Can you work these out from the model? Positions are in its coordinate system, mm. Face numbers are marked on the shaded views. A direction names the side the tool comes from. Coordinates: 2 decimals unless noted, no trailing zeros. Loops run counter-clockwise (first coordinate to the right, second up) from the corner with the lowest first, then second, coordinate; pieces in that order, holes last. Notation, with made-up numbers: M 12.25,75 L 57.25,75 A17 cw 57.25,85 Z; hole C 35,54.25 d8. An arc over 180 degrees is marked long. Answer as a JSON object with one key per item and string values. Group by question number.
Item 1: I'm going to push a flat-ended pin straight in: pin 1 Ø5 at (y, z) = (-1.5, 12) entering from +X. Where does the tip first touch, or does it pass through?
Item 2: Which directions (+Z, -Z, +X, -X, +Y, -Y) give clear straight access to the entire face, cutting with the end or side of a thin tool? Please do the marked faces 4 and 5.
Item 3: We'd pull the mould along Y, two halves only. Please class the marked faces 1, 2 and 3: +Y half, -Y half, draft (parallel to the pull), parting line (faces both ways), or undercut.
Item 4: Suppose I cut it at A-A (x = -7.5). Write out the boundary of the cut face in (y, z).
Item 5: If I drill on line 1 (X direction, y = -7, z = 3); line 2 (Y direction, x = 4.5, z = 46), over which ranges is the centre line in solid material (lowest first)?
```python
from build123d import *

# Parameters (mm, degrees)
RESSALTO_EXTRUS_O1_DEPTH = 50
PADR_OCIRCULAR1_COUNT    = 4
FILETE1_R                = 0.4


with BuildPart() as part:
    # Esboço1 → Ressalto-extrusão1 (new body)
    with BuildSketch(Plane.XY):
        with BuildLine():
            ThreePointArc((-9.317157288, 3.217157288), (-9.187387948, 3.130448187), (-9.034314575, 3.1))
            Line((-9.034314575, 3.1), (-8.9, 3.1))
            ThreePointArc((-8.9, 3.1), (-8.617157288, 3.217157288), (-8.5, 3.5))
            Line((-8.5, 3.5), (-8.5, 5.5))
            Line((-8.5, 5.5), (-6.560660172, 5.5))
            Line((-6.560660172, 5.5), (-5.064466094, 4.003805922))
            ThreePointArc((-5.064466094, 4.003805922), (-3.980602337, 2.381689178), (-3.6, 0.468272016))
            Line((-3.6, 0.468272016), (-3.6, 0))
            Line((-3.6, 0), (-2.5, 0))
            ThreePointArc((-2.5, 0), (-1.767766953, 1.767766953), (0, 2.5))
            Line((0, 2.5), (0, 3.6))
            Line((0, 3.6), (-0.468272016, 3.6))
            ThreePointArc((-0.468272016, 3.6), (-2.381689178, 3.980602337), (-4.003805922, 5.064466094))
            Line((-4.003805922, 5.064466094), (-5.5, 6.560660172))
            Line((-5.5, 6.560660172), (-5.5, 8.5))
            Line((-5.5, 8.5), (-3.5, 8.5))
            ThreePointArc((-3.5, 8.5), (-3.217157288, 8.617157288), (-3.1, 8.9))
            Line((-3.1, 8.9), (-3.1, 9.034314575))
            ThreePointArc((-3.1, 9.034314575), (-3.130448187, 9.187387948), (-3.217157288, 9.317157288))
            Line((-3.217157288, 9.317157288), (-3.782842712, 9.882842712))
            ThreePointArc((-3.782842712, 9.882842712), (-3.912612052, 9.969551813), (-4.065685425, 10))
            Line((-4.065685425, 10), (-10, 10))
            Line((-10, 10), (-10, 4.065685425))
            ThreePointArc((-10, 4.065685425), (-9.969551813, 3.912612052), (-9.882842712, 3.782842712))
            Line((-9.882842712, 3.782842712), (-9.317157288, 3.217157288))
        make_face()
    ressalto_extrus_o1 = extrude(amount=RESSALTO_EXTRUS_O1_DEPTH)

    # PadrãoCircular1: Ressalto-extrusão1 ×4 about axis
    padr_ocircular1_axis = Axis((0, 0, 0), (0, 0, 1))
    for i in range(1, PADR_OCIRCULAR1_COUNT):
        add(ressalto_extrus_o1.rotate(padr_ocircular1_axis, i * 360 / PADR_OCIRCULAR1_COUNT))

    # Filete1
    filete1_edges = [part.edges().sort_by_distance(p)[0] for p in [
        (10, -10, 25),
        (10, 10, 25),
        (-10, 10, 25),
        (-10, -10, 25),
    ]]
    fillet(filete1_edges, radius=FILETE1_R)


solid = part.part
```
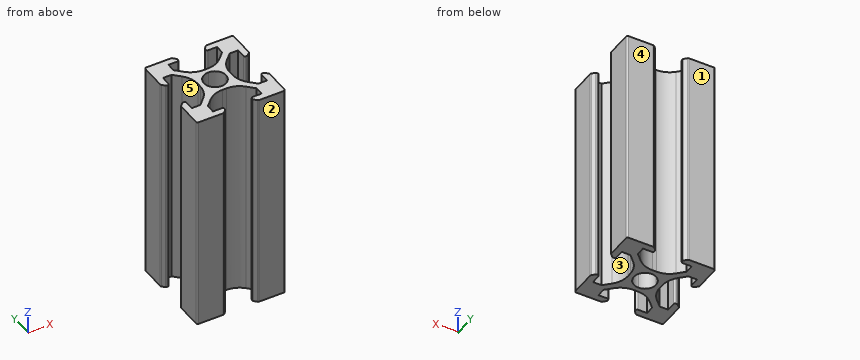
From the geometry:
{
 "1": {"pin 1": "x = 9.99"},
 "2": {"face 4": "+Z, -Z, +X, -X, +Y", "face 5": "+Z, -Z"},
 "3": {"face 1": "+Y half", "face 2": "-Y half", "face 3": "undercut"},
 "4": {"outline": "M -10,0 L -5.5,0 L -5.5,50 L -10,50 Z; M 5.5,0 L 10,0 L 10,50 L 5.5,50 Z"},
 "5": {"line 1": "-10 to -5.5, 5.5 to 10", "line 2": "-10 to -8.5, -5.56 to -3.33, 3.33 to 5.56, 8.5 to 10"}
}
